```python
from build123d import *

# Parameters (mm, degrees)
F0_W         = 19
F0_H         = 25
F1_DEPTH     = 16
F2_W         = 13.5
F2_H         = 13.5011018194
F3_DEPTH     = 50
F4_W         = 5.15
F4_H         = 10.3
F5_DEPTH     = 2.75
F6_DEPTH     = 15
F7_T1_DEPTH  = 2.4988981806
F7_T3_DEPTH  = 13.2999992773
F7_T5_DEPTH  = 13.2999992773
F7_T11_DEPTH = 21.6634917276
F7_T15_DEPTH = 25.7999992773
F7_T23_DEPTH = 21.6634917276
F7_T27_DEPTH = 25.7999992773
F7_T35_DEPTH = 22.0158699277
F7_T39_DEPTH = 25.7999992773
F7_T47_DEPTH = 25.7999992773
F7_T52_DEPTH = 22.0158699277


# Not quite as in the source:
# - a fillet or chamfer that OpenCascade refuses, or shapes differently, is made with other operations: its cross-section is extruded or revolved along the edge and cut away or added
# - a feature names something its author has since deleted; it is built from what else it names


with BuildPart() as f1:
    # F0 (on Top) → F1 (new body)
    with BuildSketch(Plane.XY):
        Rectangle(F0_W, F0_H)
    extrude(amount=F1_DEPTH)

    # F2 (on face) → F3 (cut)
    with BuildSketch(Plane.XZ.offset(12.5)):
        with Locations((0, 6.7505509097)):
            Rectangle(F2_W, F2_H)
    extrude(amount=-F3_DEPTH, mode=Mode.SUBTRACT)

    # F4 (on face) → F5 (join)
    with BuildSketch(Plane.YZ.offset(9.5)):
        Polygon((0, 16), (-17.5, 16), (-17.5, 0), (0, 0), (0, 1.4159553841), (-6.6499996386, 1.4159553841), (-6.6499996386, 14.7159546614), (0, 14.7159546614), align=None)
        Polygon((17.5, 16), (0, 16), (0, 14.7159546614), (6.6499996386, 14.7159546614), (6.6499996386, 1.4159553841), (0, 1.4159553841), (0, 0), (17.5, 0), align=None)
        with Locations((-2.575, 8.0659550227)):
            Rectangle(F4_W, F4_H)
        with Locations((2.575, 8.0659550227)):
            Rectangle(F4_W, F4_H)
        Polygon((0, 13.2159550227), (0, 14.7159546614), (-6.6499996386, 14.7159546614), (-6.6499996386, 1.4159553841), (0, 1.4159553841), (0, 2.9159550227), (-5.15, 2.9159550227), (-5.15, 13.2159550227), align=None)
        Polygon((6.6499996386, 14.7159546614), (0, 14.7159546614), (0, 13.2159550227), (5.15, 13.2159550227), (5.15, 2.9159550227), (0, 2.9159550227), (0, 1.4159553841), (6.6499996386, 1.4159553841), align=None)
    extrude(amount=-F5_DEPTH)

    # F4 (on face) → F6 (join)
    with BuildSketch(Plane.YZ.offset(9.5)):
        Polygon((0, 13.2159550227), (0, 14.7159546614), (-6.6499996386, 14.7159546614), (-6.6499996386, 1.4159553841), (0, 1.4159553841), (0, 2.9159550227), (-5.15, 2.9159550227), (-5.15, 13.2159550227), align=None)
        Polygon((6.6499996386, 14.7159546614), (0, 14.7159546614), (0, 13.2159550227), (5.15, 13.2159550227), (5.15, 2.9159550227), (0, 2.9159550227), (0, 1.4159553841), (6.6499996386, 1.4159553841), align=None)
    extrude(amount=F6_DEPTH)

    # F7: fillet of radius 5 on 6 edges, made by hand

    # F7_s2 → F7_t1 (join)
    with BuildSketch(Plane.XY.offset(13.5011018194)):
        with BuildLine():
            ThreePointArc((6.75, 17.5), (5.2855339059, 13.9644660941), (1.75, 12.5))
            Line((1.75, 12.5), (6.75, 12.5))
            Line((6.75, 12.5), (6.75, 17.5))
        make_face()
        with BuildLine():
            ThreePointArc((6.75, -17.5), (5.2855339059, -13.9644660941), (1.75, -12.5))
            Line((1.75, -12.5), (6.75, -12.5))
            Line((6.75, -12.5), (6.75, -17.5))
        make_face()
    extrude(amount=F7_T1_DEPTH)

    # F7_s4 → F7_t3 (join)
    with BuildSketch(Plane.XZ.offset(-6.6499996386)):
        with BuildLine():
            ThreePointArc((9.5, 16), (11.0537180617, 15.0479907955), (12.8453969801, 14.7159546614))
            Line((12.8453969801, 14.7159546614), (9.5, 14.7159546614))
            Line((9.5, 14.7159546614), (9.5, 16))
        make_face()
        with BuildLine():
            ThreePointArc((9.5, 0), (11.1048891295, 1.0484613517), (12.9863482602, 1.4159553841))
            Line((12.9863482602, 1.4159553841), (9.5, 1.4159553841))
            Line((9.5, 1.4159553841), (9.5, 0))
        make_face()
    extrude(amount=F7_T3_DEPTH)

    # F7_s6 → F7_t5 (join)
    with BuildSketch(Plane.XY.offset(1.4159553841)):
        with BuildLine():
            ThreePointArc((9.5, -11.6499996386), (10.9644660941, -8.1144657327), (14.5, -6.6499996386))
            Line((14.5, -6.6499996386), (9.5, -6.6499996386))
            Line((9.5, -6.6499996386), (9.5, -11.6499996386))
        make_face()
        with BuildLine():
            ThreePointArc((9.5, 11.6499996386), (10.9644660941, 8.1144657327), (14.5, 6.6499996386))
            Line((14.5, 6.6499996386), (9.5, 6.6499996386))
            Line((9.5, 6.6499996386), (9.5, 11.6499996386))
        make_face()
    extrude(amount=F7_T5_DEPTH)


with BuildPart() as f7_tool9:
    # F7_s10 → F7_t11 (new body)
    with BuildSketch(Plane.XZ.offset(-15.013492089)):
        with BuildLine():
            ThreePointArc((9.5, 16), (11.0537180617, 15.0479907955), (12.8453969801, 14.7159546614))
            Line((12.8453969801, 14.7159546614), (9.5, 14.7159546614))
            Line((9.5, 14.7159546614), (9.5, 16))
        make_face()
    extrude(amount=F7_T11_DEPTH)

    split(bisect_by=Plane.XZ.offset(-6.6499996386), keep=Keep.BOTTOM)


with BuildPart() as f7_tool13:
    # F7_s14 → F7_t15 (new body)
    with BuildSketch(Plane.XY.offset(1.4159553841)):
        with BuildLine():
            ThreePointArc((9.5, 11.6499996386), (10.9644660941, 8.1144657327), (14.5, 6.6499996386))
            Line((14.5, 6.6499996386), (9.5, 6.6499996386))
            Line((9.5, 6.6499996386), (9.5, 11.6499996386))
        make_face()
    extrude(amount=F7_T15_DEPTH)

    split(bisect_by=Plane.XY.offset(16), keep=Keep.BOTTOM)

    split(bisect_by=Plane.XY.offset(14.7159546614), keep=Keep.TOP)


with BuildPart() as f7_tool9_1:
    add(f7_tool9.part)

    # F7_t18: intersect F7_tool13
    add(f7_tool13.part, mode=Mode.INTERSECT)


with BuildPart() as f1_1:
    add(f1.part)

    # F7_t7: union F7_tool9
    add(f7_tool9_1.part)


with BuildPart() as f7_tool21:
    # F7_s22 → F7_t23 (new body)
    with BuildSketch(Plane.XZ.offset(-6.6499996386)):
        with BuildLine():
            ThreePointArc((9.5, 16), (11.0537180617, 15.0479907955), (12.8453969801, 14.7159546614))
            Line((12.8453969801, 14.7159546614), (9.5, 14.7159546614))
            Line((9.5, 14.7159546614), (9.5, 16))
        make_face()
    extrude(amount=F7_T23_DEPTH)

    split(bisect_by=Plane.XZ.offset(6.6499996386), keep=Keep.TOP)


with BuildPart() as f7_tool25:
    # F7_s26 → F7_t27 (new body)
    with BuildSketch(Plane.XY.offset(27.2159546614)):
        with BuildLine():
            ThreePointArc((9.5, -11.6499996386), (10.9644660941, -8.1144657327), (14.5, -6.6499996386))
            Line((14.5, -6.6499996386), (9.5, -6.6499996386))
            Line((9.5, -6.6499996386), (9.5, -11.6499996386))
        make_face()
    extrude(amount=-F7_T27_DEPTH)

    split(bisect_by=Plane.XY.offset(16), keep=Keep.BOTTOM)

    split(bisect_by=Plane.XY.offset(14.7159546614), keep=Keep.TOP)


with BuildPart() as f7_tool21_1:
    add(f7_tool21.part)

    # F7_t30: intersect F7_tool25
    add(f7_tool25.part, mode=Mode.INTERSECT)


with BuildPart() as f1_2:
    add(f1_1.part)

    # F7_t19: union F7_tool21
    add(f7_tool21_1.part)


with BuildPart() as f7_tool33:
    # F7_s34 → F7_t35 (new body)
    with BuildSketch(Plane.XZ.offset(15.365870289)):
        with BuildLine():
            ThreePointArc((9.5, 0), (11.1048891295, 1.0484613517), (12.9863482602, 1.4159553841))
            Line((12.9863482602, 1.4159553841), (9.5, 1.4159553841))
            Line((9.5, 1.4159553841), (9.5, 0))
        make_face()
    extrude(amount=-F7_T35_DEPTH)

    split(bisect_by=Plane.XZ.offset(6.6499996386), keep=Keep.TOP)


with BuildPart() as f7_tool37:
    # F7_s38 → F7_t39 (new body)
    with BuildSketch(Plane.XY.offset(14.7159546614)):
        with BuildLine():
            ThreePointArc((9.5, -11.6499996386), (10.9644660941, -8.1144657327), (14.5, -6.6499996386))
            Line((14.5, -6.6499996386), (9.5, -6.6499996386))
            Line((9.5, -6.6499996386), (9.5, -11.6499996386))
        make_face()
    extrude(amount=-F7_T39_DEPTH)

    split(bisect_by=Plane.XY, keep=Keep.TOP)

    split(bisect_by=Plane.XY.offset(1.4159553841), keep=Keep.BOTTOM)


with BuildPart() as f7_tool33_1:
    add(f7_tool33.part)

    # F7_t42: intersect F7_tool37
    add(f7_tool37.part, mode=Mode.INTERSECT)


with BuildPart() as f1_3:
    add(f1_2.part)

    # F7_t31: union F7_tool33
    add(f7_tool33_1.part)


with BuildPart() as f7_tool45:
    # F7_s46 → F7_t47 (new body)
    with BuildSketch(Plane.XY.offset(-11.0840446159)):
        with BuildLine():
            ThreePointArc((9.5, 11.6499996386), (10.9644660941, 8.1144657327), (14.5, 6.6499996386))
            Line((14.5, 6.6499996386), (9.5, 6.6499996386))
            Line((9.5, 6.6499996386), (9.5, 11.6499996386))
        make_face()
    extrude(amount=F7_T47_DEPTH)

    split(bisect_by=Plane.XY, keep=Keep.TOP)

    split(bisect_by=Plane.XY.offset(1.4159553841), keep=Keep.BOTTOM)


with BuildPart() as f7_tool50:
    # F7_s51 → F7_t52 (new body)
    with BuildSketch(Plane.XZ.offset(6.6499996386)):
        with BuildLine():
            ThreePointArc((9.5, 0), (11.1048891295, 1.0484613517), (12.9863482602, 1.4159553841))
            Line((12.9863482602, 1.4159553841), (9.5, 1.4159553841))
            Line((9.5, 1.4159553841), (9.5, 0))
        make_face()
    extrude(amount=-F7_T52_DEPTH)

    split(bisect_by=Plane.XZ.offset(-6.6499996386), keep=Keep.BOTTOM)


with BuildPart() as f7_tool45_1:
    add(f7_tool45.part)

    # F7_t54: intersect F7_tool50
    add(f7_tool50.part, mode=Mode.INTERSECT)


with BuildPart() as f1_4:
    add(f1_3.part)

    # F7_t43: union F7_tool45
    add(f7_tool45_1.part)


solid = f1_4.part
```
Geometry check sheet. Reference: the model listing, model coordinates, mm. A direction names the side the tool comes from. Coordinates: 2 decimals unless noted, no trailing zeros. Loops run counter-clockwise (first coordinate to the right, second up) from the corner with the lowest first, then second, coordinate; pieces in that order, holes last.
Item 1: Sectioned sample at B-B, the plane z = 11.25. Record the boundary of the cut face in (x, y).
Item 2: Sectioned sample at D-D, the plane x = 1. Record the boundary of the cut face in (y, z), then the cut area to 3 significant figures.
Item 3: Sectioned sample at A-A, the plane x = 15.5. Record the boundary of the cut face in (y, z), then the cut area to 3 significant figures.
Item 4: Go/stop test with flat-tipped pins: pin 1 Ø4 at (x, z) = (17.5, 5.5) entering from -Y; pin 2 Ø11.5 at (x, y) = (15, 1) entering from -Z; pin 3 Ø4 at (y, z) = (0.5, 5.5) entering from +X; pin 4 Ø13 at (x, y) = (17.5, 0.5) entering from +Z. Record where each tip stops, or that it passes through.
Item 5: Thickness scan on line 1 (Y direction, x = 13, z = 9); line 2 (X direction, y = 6, z = 6.25); line 3 (X direction, y = -5, z = 3.75). Record the ranges inside material, lowest first.
Item 6: Release check for a two-part mould opening along Y. For faces 5 (the face through (-7, -12.5, 10)), 6 (the face through (9.5, 0, 8)), 7 (the face through (-9.5, 0, 8)), 8 (the face through (17, -5.15, 8)) record: released by +Y, released by -Y, zero draft, split by the parting line, or undercut.
Item 7: Sectioned sample at C-C, the plane y = 4. Record the boundary of the cut face in (x, z).
Item 8: Access from +Z, -Z, +X, -X, +Y, -Y to the whole of each face (thin tool, end or side, straight path). Record for faces 1 (the face through (17, 0, 2.916)), 2 (the face through (9.5, 15, 8)), 3 (the face through (-7, 12.5, 10)), 4 (the face through (19, 0, 14.716)).
Check result:
1. outline: (-9.5, -12.5) - (-6.75, -12.5) - (-6.75, 12.5) - (-9.5, 12.5) - close; (6.75, -17.5) - (9.5, -17.5) - (9.5, -11.65) arc R5 cw to (14.5, -6.65) - (24.5, -6.65) - (24.5, -5.15) - (9.5, -5.15) - (9.5, 5.15) - (24.5, 5.15) - (24.5, 6.65) - (14.5, 6.65) arc R5 cw to (9.5, 11.65) - (9.5, 17.5) - (6.75, 17.5) - close
2. outline: (-12.5, 13.5) - (12.5, 13.5) - (12.5, 16) - (-12.5, 16) - close
2. area: 62.5 mm2
3. outline: (-6.65, 1.42) - (6.65, 1.42) - (6.65, 14.72) - (-6.65, 14.72) - close; hole (-5.15, 2.92) - (5.15, 2.92) - (5.15, 13.22) - (-5.15, 13.22) - close
3. area: 70.8 mm2
4. pin 1: stops at y = -6.65
4. pin 2: stops at z = 0
4. pin 3: stops at x = 9.5
4. pin 4: stops at z = 15.07
5. line 1: y = -6.88 to -5.15, 5.15 to 6.88
5. line 2: x = -9.5 to -6.75, 6.75 to 24.5
5. line 3: x = -9.5 to -6.75, 6.75 to 9.5
6. face 5: released by -Y
6. face 6: undercut
6. face 7: zero draft
6. face 8: undercut
7. outline: (-9.5, 0) - (-6.75, 0) - (-6.75, 13.5) - (6.75, 13.5) - (6.75, 0) - (9.5, 0) arc R5 cw to (12.99, 1.42) - (24.5, 1.42) - (24.5, 2.92) - (9.5, 2.92) - (9.5, 13.22) - (24.5, 13.22) - (24.5, 14.72) - (12.85, 14.72) arc R5 cw to (9.5, 16) - (-9.5, 16) - close
8. face 1: +X
8. face 2: +Z, -Z, +X, +Y
8. face 3: +Z, -Z, -X, +Y
8. face 4: +Z, +X, +Y, -Y
